from build123d import *

# Parameters (mm, degrees)
BOSS_EXTRUDE1_DEPTH              = 1.68939972
F_2_9_2_9_DIAMETER_HOLE1_D       = 2.89999928
F_2_9_2_9_DIAMETER_HOLE1_DEPTH   = 1.68939972
HOLE1_D                          = 0.8999982
HOLE1_DEPTH                      = 1.68939972
LPATTERN1_COUNT                  = 5
LPATTERN1_PITCH                  = 2.54
HOLE2_D                          = 0.999998
HOLE2_DEPTH                      = 1.68939972
LPATTERN2_COUNT                  = 2
LPATTERN2_PITCH                  = 2.54
LPATTERN2_COUNT_DIR2             = 10
LPATTERN2_PITCH_DIR2             = 2.54
HOLE3_D                          = 1.1999976
HOLE3_DEPTH                      = 1.68939972
LPATTERN3_COUNT                  = 2
LPATTERN3_PITCH                  = 2.540004919
HOLE4_D                          = 1.1999976
HOLE4_DEPTH                      = 1.68939972
LPATTERN4_COUNT                  = 2
LPATTERN4_PITCH                  = 2.540004919
F_2_9_2_9_DIAMETER_HOLE2_D       = 2.89999928
F_2_9_2_9_DIAMETER_HOLE2_DEPTH   = 1.68939972
F_2_9_2_9_DIAMETER_HOLE3_D       = 2.89999928
F_2_9_2_9_DIAMETER_HOLE3_DEPTH   = 1.68939972
F_0_85_0_85_DIAMETER_HOLE1_D     = 0.85000084
F_0_85_0_85_DIAMETER_HOLE1_DEPTH = 1.68939972
LPATTERN5_COUNT                  = 2
LPATTERN5_PITCH                  = 6.80000164
HOLE5_D                          = 0.7999984
HOLE5_DEPTH                      = 1.68939972
LPATTERN6_COUNT                  = 3
LPATTERN6_PITCH                  = 3.99999962
LPATTERN6_COUNT_DIR2             = 2
LPATTERN6_PITCH_DIR2             = 2.50000008
F_2_9_2_9_DIAMETER_HOLE4_D       = 2.89999928
F_2_9_2_9_DIAMETER_HOLE4_DEPTH   = 1.68939972
HOLE6_D                          = 1.1999976
HOLE6_DEPTH                      = 1.68939972
LPATTERN7_COUNT                  = 2
LPATTERN7_PITCH                  = 12.200001
F_2_9_2_9_DIAMETER_HOLE5_D       = 2.89999928
F_2_9_2_9_DIAMETER_HOLE5_DEPTH   = 1.68939972


with BuildPart() as part:
    # Sketch1 → Boss-Extrude1 (new body)
    with BuildSketch(Plane.XY.offset(1.68939972)):
        with BuildLine():
            Line((87.300003052, 25.399999619), (87.300003052, 29.399999619))
            ThreePointArc((87.300003052, 29.399999619), (87.592896271, 30.1071064), (88.300003052, 30.399999619))
            Line((88.300003052, 30.399999619), (101.5, 30.399999619))
            ThreePointArc((101.5, 30.399999619), (102.207106781, 30.1071064), (102.5, 29.399999619))
            Line((102.5, 29.399999619), (102.5, 25.399999619))
            Line((102.5, 25.399999619), (124.900001526, 25.399999619))
            Line((124.900001526, 25.399999619), (124.900001526, 99.5))
            Line((124.900001526, 99.5), (33.400001526, 99.5))
            Line((33.400001526, 99.5), (33.400001526, 93.949998856))
            ThreePointArc((33.400001526, 93.949998856), (32.374874701, 91.475123773), (29.899999619, 90.449996948))
            Line((29.899999619, 90.449996948), (25.399999619, 90.449996948))
            Line((25.399999619, 90.449996948), (25.399999619, 34.450000763))
            Line((25.399999619, 34.450000763), (29.899999619, 34.450000763))
            ThreePointArc((29.899999619, 34.450000763), (32.374874701, 33.424873938), (33.400001526, 30.949998856))
            Line((33.400001526, 30.949998856), (33.400001526, 25.399999619))
            Line((33.400001526, 25.399999619), (87.300003052, 25.399999619))
        make_face()
    extrude(amount=-BOSS_EXTRUDE1_DEPTH)

    # 2.9 _2.9_ Diameter Hole1
    with Locations(Plane(origin=(0, 0, 0), x_dir=(-1, 0, 0), z_dir=(0, 0, -1))):
        with Locations((-122.39998888, 62.44998432)):
            Hole(F_2_9_2_9_DIAMETER_HOLE1_D / 2, depth=F_2_9_2_9_DIAMETER_HOLE1_DEPTH)

    # Hole1
    with Locations(Plane(origin=(0, 0, 0), x_dir=(-1, 0, 0), z_dir=(0, 0, -1))):
        with Locations((-112.52199746, 94.4230014)):
            hole1 = Hole(HOLE1_D / 2, depth=HOLE1_DEPTH)

    # LPattern1: Hole1 ×5
    with Locations(*[(0, -i * LPATTERN1_PITCH, 0) for i in range(1, LPATTERN1_COUNT)]):
        add(hole1, mode=Mode.SUBTRACT)

    # Hole2
    with Locations(Plane(origin=(0, 0, 0), x_dir=(-1, 0, 0), z_dir=(0, 0, -1))):
        with Locations((-113.284, 38.227)):
            hole2 = Hole(HOLE2_D / 2, depth=HOLE2_DEPTH)

    # LPattern2: Hole2 2 × 10
    with Locations(*[(i * LPATTERN2_PITCH, j * LPATTERN2_PITCH_DIR2, 0) for i in range(LPATTERN2_COUNT) for j in range(LPATTERN2_COUNT_DIR2) if (i, j) != (0, 0)]):
        add(hole2, mode=Mode.SUBTRACT)

    # Hole3
    with Locations(Plane(origin=(0, 0, 0), x_dir=(-1, 0, 0), z_dir=(0, 0, -1))):
        with Locations((-109.47899872, 79.121)):
            hole3 = Hole(HOLE3_D / 2, depth=HOLE3_DEPTH)

    # LPattern3: Hole3 ×2
    with Locations(*[Vector(-0.001967996, -0.999998063, 0) * (i * LPATTERN3_PITCH) for i in range(1, LPATTERN3_COUNT)]):
        add(hole3, mode=Mode.SUBTRACT)

    # Hole4
    with Locations(Plane(origin=(0, 0, 0), x_dir=(-1, 0, 0), z_dir=(0, 0, -1))):
        with Locations((-109.47899872, 68.961)):
            hole4 = Hole(HOLE4_D / 2, depth=HOLE4_DEPTH)

    # LPattern4: Hole4 ×2
    with Locations(*[Vector(-0.001967996, -0.999998063, 0) * (i * LPATTERN4_PITCH) for i in range(1, LPATTERN4_COUNT)]):
        add(hole4, mode=Mode.SUBTRACT)

    # 2.9 _2.9_ Diameter Hole2
    with Locations(Plane(origin=(0, 0, 0), x_dir=(-1, 0, 0), z_dir=(0, 0, -1))):
        with Locations((-46.1999838, 90.44998928)):
            Hole(F_2_9_2_9_DIAMETER_HOLE2_D / 2, depth=F_2_9_2_9_DIAMETER_HOLE2_DEPTH)

    # 2.9 _2.9_ Diameter Hole3
    with Locations(Plane(origin=(0, 0, 0), x_dir=(-1, 0, 0), z_dir=(0, 0, -1))):
        with Locations((-33.399984, 84.94998504)):
            Hole(F_2_9_2_9_DIAMETER_HOLE3_D / 2, depth=F_2_9_2_9_DIAMETER_HOLE3_DEPTH)

    # 0.85 _0.85_ Diameter Hole1
    with Locations(Plane(origin=(0, 0, 0), x_dir=(-1, 0, 0), z_dir=(0, 0, -1))):
        with Locations((-27.25008266, 65.84998768)):
            f_0_85_0_85_diameter_hole1 = Hole(F_0_85_0_85_DIAMETER_HOLE1_D / 2, depth=F_0_85_0_85_DIAMETER_HOLE1_DEPTH)

    # LPattern5: 0.85 _0.85_ Diameter Hole1 ×2
    with Locations(*[(0, -i * LPATTERN5_PITCH, 0) for i in range(1, LPATTERN5_COUNT)]):
        add(f_0_85_0_85_diameter_hole1, mode=Mode.SUBTRACT)

    # Hole5
    with Locations(Plane(origin=(0, 0, 0), x_dir=(-1, 0, 0), z_dir=(0, 0, -1))):
        with Locations((-90.29998196, 36.04998632)):
            hole5 = Hole(HOLE5_D / 2, depth=HOLE5_DEPTH)

    # LPattern6: Hole5 3 × 2
    with Locations(*[(i * LPATTERN6_PITCH, -j * LPATTERN6_PITCH_DIR2, 0) for i in range(LPATTERN6_COUNT) for j in range(LPATTERN6_COUNT_DIR2) if (i, j) != (0, 0)]):
        add(hole5, mode=Mode.SUBTRACT)

    # 2.9 _2.9_ Diameter Hole4
    with Locations(Plane(origin=(0, 0, 0), x_dir=(-1, 0, 0), z_dir=(0, 0, -1))):
        with Locations((-46.1999838, 34.44998952)):
            Hole(F_2_9_2_9_DIAMETER_HOLE4_D / 2, depth=F_2_9_2_9_DIAMETER_HOLE4_DEPTH)

    # Hole6
    with Locations(Plane(origin=(0, 0, 0), x_dir=(-1, 0, 0), z_dir=(0, 0, -1))):
        with Locations((-88.19998108, 34.79998628)):
            hole6 = Hole(HOLE6_D / 2, depth=HOLE6_DEPTH)

    # LPattern7: Hole6 ×2
    with Locations(*[(i * LPATTERN7_PITCH, 0, 0) for i in range(1, LPATTERN7_COUNT)]):
        add(hole6, mode=Mode.SUBTRACT)

    # 2.9 _2.9_ Diameter Hole5
    with Locations(Plane(origin=(0, 0, 0), x_dir=(-1, 0, 0), z_dir=(0, 0, -1))):
        with Locations((-33.399984, 39.9499836)):
            Hole(F_2_9_2_9_DIAMETER_HOLE5_D / 2, depth=F_2_9_2_9_DIAMETER_HOLE5_DEPTH)


solid = part.part
The listing builds one solid part. Answer for the finished solid, in the listing's coordinates (mm). Coordinates: 2 decimals unless noted, no trailing zeros. Write item = value, one per line. Start each with the question number.
1) The mould has two halves that part along Y. Classify faces 1 (the face through (122.086, 61.034, 0.857)), 2 (the face through (32.4, 91.5, 0.9)), 3 (the face through (74, 63, 0)), 4 (the face through (32.3, 33.5, 0.9)): released by +Y, released by -Y, zero draft, split by the parting line, or undercut.
2) Given pin 1 Ø4 at (x, y) = (33.4, 39.95) entering from -Z; pin 2 Ø0.5 at (y, z) = (27.5, 1) entering from -X, each flat-ended and moving along its own axis, determine where each tip first touches the part or whether it passes through.
3) A cutting plane is placed at A-A (z = 1.1). Count the separate pieces of the cut face and the enclosed holes in it, then the cut area to 4 significant figures.
4) Straight lines are drawn through the part: line 1 (X direction, y = 69, z = 0.5); line 2 (Y direction, x = 45.5, z = 0.8); line 3 (Y direction, x = 95, z = 0.35). For each, find the intervals that lie inside material, in ascending order. Write a range as from..to.
Responses:
q1.face_1 = undercut
q1.face_2 = released by +Y
q1.face_3 = zero draft
q1.face_4 = released by -Y
q2.pin_1 = 0
q2.pin_2 = 33.4
q3.separate_pieces = 1
q3.enclosed_holes = 44
q3.area = 7,095 mm²
q4.line_1 = 25.4..108.88, 110.08..124.9
q4.line_2 = 25.4..33.18, 35.72..89.18, 91.72..99.5
q4.line_3 = 30.4..99.5
